Verification items for the finished model (mm, model axes). A direction names the side the tool comes from. Coordinates: 2 decimals unless noted, no trailing zeros. Loops run counter-clockwise (first coordinate to the right, second up) from the corner with the lowest first, then second, coordinate; pieces in that order, holes last. Notation, with made-up numbers: (34, -10.75) - (47, -10.75) arc R32 ccw to (47, 19.25) - close; hole circle Ø1 at (51, 17.5). An arc over 180 degrees is marked (long way). One line per item, written item: value. Start each with the question number.
(1) Set-up check for faces 4 (the face through (-107.7, 143.7, 3)), 5 (the face through (-241, 52, 3)), 6 (the face through (-204, 145, 3)), 7 (the face through (-334, 11, 3)): record each of +Z, -Z, +X, -X, +Y, -Y from which the full face is reachable in a straight line by a thin tool's end or side.
(2) Section check A-A (y = 71). Record the boundary of the cut face in (x, z), plus the area to 3 significant figures.
(3) Draft check along X on faces 1 (the face through (-334, 83, 3)), 2 (the face through (-310, 32, 3)), 3 (the face through (-337, 18, 3)). Enter one of: +X half, -X half, draft (parallel to the pull), parting line (faces both ways), or undercut.
(4) Gauge pin test, flat ends, axial feed: P1, Ø8, axis at x = -109, y = 145, coming from the +Z side; P2, Ø1.8, axis at y = 12.5, z = 3.5, coming from the -X side; P3, Ø1.8, axis at x = -284, z = 1.5, coming from the +Y side; P4, Ø3, axis at y = -4.5, z = 2, coming from the -X side. Record the tip position at first contact, or that the pin passes through.
(5) Section check C-C (x = -159.5). Record the boundary of the cut face in (y, z).
(6) Section check B-B (y = 42.5). Record the boundary of the cut face in (x, z), plus the area to 3 significant figures.
(7) Thickness scan on probe 1 along Y at (x, z) = (-165, 4.8); probe 2 along X at (y, z) = (145, 0.7); probe 3 along Y at (x, z) = (-293, 4.85). Record the ranges inside material, lowest first. Write a range as [from, to].
```python
from build123d import *

# Parameters (mm, degrees)
ESQUISSE1_W              = 340
ESQUISSE1_H              = 148
BOSS_EXTRU_1_DEPTH       = 6
ESQUISSE2_W              = 6
ESQUISSE2_H              = 28
ESQUISSE2_H_2            = 18
ESQUISSE2_W_2            = 68
ESQUISSE2_H_3            = 6
ESQUISSE2_H_4            = 30
ENL_V_MAT_EXTRU_1_DEPTH  = 6
ESQUISSE3_W              = 6
ESQUISSE3_H              = 20
ESQUISSE3_W_2            = 30
ESQUISSE3_H_2            = 25
ESQUISSE3_W_3            = 20
ESQUISSE3_H_3            = 6
ENL_V_MAT_EXTRU_2_DEPTH  = 10
ESQUISSE4_R              = 1.5
ESQUISSE4_W              = 10
ESQUISSE4_H              = 6
ENL_V_MAT_EXTRU_3_DEPTH  = 10
ESQUISSE7_W              = 328
ESQUISSE7_H              = 6
BOSS_EXTRU_2_DEPTH       = 17
ESQUISSE8_R              = 1.5
ESQUISSE8_W              = 20
ESQUISSE8_H              = 20
ENL_V_MAT_EXTRU_5_DEPTH  = 371.863856422
ESQUISSE9_R              = 2.995
ESQUISSE9_R_2            = 3
ENL_V_MAT_EXTRU_8_DEPTH  = 3
ESQUISSE10_W             = 130.302032554
ESQUISSE10_H             = 194.077332213
ENL_V_MAT_EXTRU_9_DEPTH  = 371.863856422
ESQUISSE11_W             = 6
ESQUISSE11_H             = 30
ENL_V_MAT_EXTRU_10_DEPTH = 3


with BuildPart() as part:
    # Esquisse1 → Boss.-Extru.1 (new body)
    with BuildSketch(Plane.XY):
        with Locations((-170, 74)):
            Rectangle(ESQUISSE1_W, ESQUISSE1_H)
    extrude(amount=BOSS_EXTRU_1_DEPTH)

    # Esquisse2 → Enlèv. mat.-Extru.1 (cut)
    with BuildSketch(Plane.XY.offset(6)):
        Polygon((-272, 142), (-334, 142), (-334, 48), (-340, 48), (-340, 148), (-272, 148), align=None)
        Polygon((0, 148), (0, 118), (-6, 118), (-6, 142), (-68, 142), (-68, 148), align=None)
        with Locations((-3, 14)):
            Rectangle(ESQUISSE2_W, ESQUISSE2_H)
        with Locations((-337, 9)):
            Rectangle(ESQUISSE2_W, ESQUISSE2_H_2)
        with Locations((-170, 145)):
            Rectangle(ESQUISSE2_W_2, ESQUISSE2_H_3)
        with Locations((-3, 73)):
            Rectangle(ESQUISSE2_W, ESQUISSE2_H_4)
    extrude(amount=-ENL_V_MAT_EXTRU_1_DEPTH, mode=Mode.SUBTRACT)

    # Esquisse3 → Enlèv. mat.-Extru.2 (cut)
    with BuildSketch(Plane.XY.offset(6)):
        with Locations((-241, 42)):
            Rectangle(ESQUISSE3_W, ESQUISSE3_H)
        with Locations((-241, 102)):
            Rectangle(ESQUISSE3_W, ESQUISSE3_H)
        with Locations((-288.5, 70.5)):
            Rectangle(ESQUISSE3_W, ESQUISSE3_H)
        with Locations((-319, 129.5)):
            Rectangle(ESQUISSE3_W_2, ESQUISSE3_H_2)
        with Locations((-310, 105)):
            Rectangle(ESQUISSE3_W_3, ESQUISSE3_H_3)
        with Locations((-310, 29)):
            Rectangle(ESQUISSE3_W_3, ESQUISSE3_H_3)
        with Locations((-67, 102)):
            Rectangle(ESQUISSE3_W, ESQUISSE3_H)
    extrude(amount=-ENL_V_MAT_EXTRU_2_DEPTH, mode=Mode.SUBTRACT)

    # Esquisse4 → Enlèv. mat.-Extru.3 (cut)
    with BuildSketch(Plane.XY.offset(6)):
        with Locations((-151.5, 121.6)):
            Circle(ESQUISSE4_R)
        with Locations((-151.5, 5)):
            Circle(ESQUISSE4_R)
        with Locations((-169, 121.6)):
            Rectangle(ESQUISSE4_W, ESQUISSE4_H)
        with Locations((-134, 121.6)):
            Rectangle(ESQUISSE4_W, ESQUISSE4_H)
        with Locations((-134, 5)):
            Rectangle(ESQUISSE4_W, ESQUISSE4_H)
        with Locations((-169, 5)):
            Rectangle(ESQUISSE4_W, ESQUISSE4_H)
    extrude(amount=-ENL_V_MAT_EXTRU_3_DEPTH, mode=Mode.SUBTRACT)

    # Esquisse7 → Boss.-Extru.2 (add)
    with BuildSketch(Plane.XZ):
        with Locations((-170, 3)):
            Rectangle(ESQUISSE7_W, ESQUISSE7_H)
    extrude(amount=BOSS_EXTRU_2_DEPTH)

    # Esquisse8 → Enlèv. mat.-Extru.5 (cut, through all)
    with BuildSketch(Plane.XY.offset(6)):
        with Locations((-75, 145)):
            Circle(ESQUISSE8_R)
        with Locations((-129, 145)):
            Circle(ESQUISSE8_R)
        with Locations((-109, 145)):
            Circle(ESQUISSE8_R)
        with Locations((-3, 111)):
            Circle(ESQUISSE8_R)
        with Locations((-3, 95)):
            Circle(ESQUISSE8_R)
        with Locations((-3, 51)):
            Circle(ESQUISSE8_R)
        with Locations((-3, 35)):
            Circle(ESQUISSE8_R)
        with Locations((-122, 121.6)):
            Circle(ESQUISSE8_R)
        with Locations((-181, 121.6)):
            Circle(ESQUISSE8_R)
        with Locations((-122, 5)):
            Circle(ESQUISSE8_R)
        with Locations((-181, 5)):
            Circle(ESQUISSE8_R)
        with Locations((-211, 145)):
            Circle(ESQUISSE8_R)
        with Locations((-241, 145)):
            Circle(ESQUISSE8_R)
        with Locations((-241, 122)):
            Circle(ESQUISSE8_R)
        with Locations((-241, 82)):
            Circle(ESQUISSE8_R)
        with Locations((-241, 62)):
            Circle(ESQUISSE8_R)
        with Locations((-241, 22)):
            Circle(ESQUISSE8_R)
        with Locations((-241, -7)):
            Circle(ESQUISSE8_R)
        with Locations((-288.5, 87.5)):
            Circle(ESQUISSE8_R)
        with Locations((-288.5, 53.5)):
            Circle(ESQUISSE8_R)
        with Locations((-293, 105)):
            Circle(ESQUISSE8_R)
        with Locations((-327, 105)):
            Circle(ESQUISSE8_R)
        with Locations((-293, 29)):
            Circle(ESQUISSE8_R)
        with Locations((-327, 29)):
            Circle(ESQUISSE8_R)
        with Locations((-337, 33)):
            Circle(ESQUISSE8_R)
        with Locations((-324, -7)):
            Rectangle(ESQUISSE8_W, ESQUISSE8_H)
    extrude(amount=-ENL_V_MAT_EXTRU_5_DEPTH, mode=Mode.SUBTRACT)

    # Esquisse9 → Enlèv. mat.-Extru.8 (cut)
    with BuildSketch(Plane.XY.offset(6)):
        with Locations((-337, 33)):
            Circle(ESQUISSE9_R)
        with Locations((-327, 29)):
            Circle(ESQUISSE9_R_2)
        with Locations((-293, 29)):
            Circle(ESQUISSE9_R_2)
        with Locations((-288.5, 53.5)):
            Circle(ESQUISSE9_R_2)
        with Locations((-288.5, 87.5)):
            Circle(ESQUISSE9_R_2)
        with Locations((-293, 105)):
            Circle(ESQUISSE9_R_2)
        with Locations((-327, 105)):
            Circle(ESQUISSE9_R_2)
        with Locations((-241, 145)):
            Circle(ESQUISSE9_R)
        with Locations((-241, 122)):
            Circle(ESQUISSE9_R)
        with Locations((-241, 82)):
            Circle(ESQUISSE9_R)
        with Locations((-241, 62)):
            Circle(ESQUISSE9_R_2)
        with Locations((-241, 22)):
            Circle(ESQUISSE9_R_2)
        with Locations((-241, -7)):
            Circle(ESQUISSE9_R_2)
        with Locations((-211, 145)):
            Circle(ESQUISSE9_R)
        with Locations((-181, 121.6)):
            Circle(ESQUISSE9_R)
        with Locations((-151.5, 121.6)):
            Circle(ESQUISSE9_R)
        with Locations((-129, 145)):
            Circle(ESQUISSE9_R)
        with Locations((-122, 121.6)):
            Circle(ESQUISSE9_R)
        with Locations((-109, 145)):
            Circle(ESQUISSE9_R)
        with Locations((-122, 5)):
            Circle(ESQUISSE9_R)
        with Locations((-151.5, 5)):
            Circle(ESQUISSE9_R)
        with Locations((-181, 5)):
            Circle(ESQUISSE9_R)
        with Locations((-75, 145)):
            Circle(ESQUISSE9_R)
        with Locations((-3, 111)):
            Circle(ESQUISSE9_R)
        with Locations((-3, 95)):
            Circle(ESQUISSE9_R)
        with Locations((-3, 51)):
            Circle(ESQUISSE9_R)
        with Locations((-3, 35)):
            Circle(ESQUISSE9_R)
    extrude(amount=-ENL_V_MAT_EXTRU_8_DEPTH, mode=Mode.SUBTRACT)

    # Esquisse10 → Enlèv. mat.-Extru.9 (cut, through all)
    with BuildSketch(Plane.XY.offset(6)):
        with Locations((-38.848983723, 50.961333893)):
            Rectangle(ESQUISSE10_W, ESQUISSE10_H)
    extrude(amount=-ENL_V_MAT_EXTRU_9_DEPTH, mode=Mode.SUBTRACT)

    # Esquisse11 → Enlèv. mat.-Extru.10 (cut)
    with BuildSketch(Plane.XY.offset(6)):
        with Locations((-107, 67)):
            Rectangle(ESQUISSE11_W, ESQUISSE11_H)
    extrude(amount=-ENL_V_MAT_EXTRU_10_DEPTH, mode=Mode.SUBTRACT)


solid = part.part
```
Responses:
1. face 4: +Z
1. face 5: +Z, -Z
1. face 6: +Z, -Z, +Y
1. face 7: +Z, -Z, -X, -Y
2. outline: (-334, 0) - (-291.5, 0) - (-291.5, 6) - (-334, 6) - close; (-285.5, 0) - (-104, 0) - (-104, 3) - (-110, 3) - (-110, 6) - (-285.5, 6) - close
2. area: 1,330 mm²
3. face 1: -X half
3. face 2: undercut
3. face 3: draft
4. P1: stops at z = 6
4. P2: stops at x = -334
4. P3: stops at y = 142
4. P4: stops at x = -314
5. outline: (-17, 0) - (142, 0) - (142, 6) - (-17, 6) - close
6. outline: (-340, 0) - (-244, 0) - (-244, 6) - (-340, 6) - close; (-238, 0) - (-104, 0) - (-104, 6) - (-238, 6) - close
6. area: 1,380 mm²
7. probe 1: y = [-17, 2], [8, 118.6], [124.6, 142]
7. probe 2: x = [-272, -242.5], [-239.5, -212.5], [-209.5, -204], [-136, -130.5], [-127.5, -110.5], [-107.5, -104]
7. probe 3: y = [-17, 26], [32, 102], [108, 142]
